Geometry check sheet. Reference: the model listing, model coordinates, mm. A direction names the side the tool comes from. Give positions to 0.01 mm unless a question says otherwise; leave off trailing zeros. Write each loop counter-clockwise with the first axis right and the second up, starting at its lowest first coordinate (ties: lowest second). Pieces come first, ordered by that corner, then holes.
(1) Depth check by flat-ended pin: P1, Ø5, axis at x = -40, z = -35, coming from the -Y side; P2, Ø6, axis at y = 19.5, z = -37.5, coming from the -X side; P3, Ø7, axis at x = 40, z = 35, coming from the +Y side. Enter the tip coordinate at first touch or a pass-through.
(2) Mould release check, pull along Z, two halves, no side actions. Record for faces 1 (the flat face through (-1, 15, 50)), 2 (the cylindrical face through (37.973, 1.521, 33.141)), 3 (the flat face through (-45, 1, -1)): +Z half, -Z half, draft (parallel to the pull), parting line (faces both ways), or undercut.
(3) Cross-section at D-D (x = 39). Record the boundary of the cut face in (y, z).
(4) Cross-section at B-B (z = -35). Record the boundary of the cut face in (x, y), and give its area (3 significant figures).
(5) Cross-section at C-C (z = -20.5). Record the boundary of the cut face in (x, y), and give its area (3 significant figures).
(6) Tool access check on faces 4 (the flat face through (35, 16, 1)), 5 (the cylindrical face through (-42.027, 1.521, 33.141)), 6 (the flat face through (-35, 16, 1)). Record the directions out of +Z, -Z, +X, -X, +Y, -Y that give a thin tool (end or side, any length) a straight path to the whole face; none if there is none.
(7) Cross-section at A-A (x = -40). Record the boundary of the cut face in (y, z), and give its area (3 significant figures).
(8) Thickness scan on line 1 along X through (y, z) = (1.8, -35); line 2 along Z through (x, y) = (-40, 1); line 3 along X through (y, z) = (21.75, -28). Record the ranges inside material, lowest first.
```python
from build123d import *

# Parameters (mm, degrees)
SKETCH1_W                = 70
SKETCH1_H                = 100
BOSS_EXTRUDE1_DEPTH      = 30
BOSS_EXTRUDE3_DEPTH      = 3
M5_CLEARANCE_SLOT1_D     = 5.5
M5_CLEARANCE_SLOT1_DEPTH = 22.25
M5_CLEARANCE_SLOT1_TIP   = 1.652366702


with BuildPart() as part:
    # Sketch1 → Boss-Extrude1 (new body)
    with BuildSketch(Plane(origin=(0, 0, 0), x_dir=(1, 0, 0), z_dir=(0, 1, 0))):
        Rectangle(SKETCH1_W, SKETCH1_H)
    extrude(amount=BOSS_EXTRUDE1_DEPTH)

    # Sketch1<4> → Boss-Extrude3 (add)
    with BuildSketch(Plane(origin=(0, 0, 0), x_dir=(1, 0, 0), z_dir=(0, 1, 0))):
        Polygon((-35, -50), (-35, 50), (-45, 50), (-45, 35), (-45, -35), (-45, -50), align=None)
        Polygon((45, 35), (45, 50), (35, 50), (35, -50), (45, -50), (45, -35), align=None)
    extrude(amount=BOSS_EXTRUDE3_DEPTH)

    # M5 Clearance Slot1
    with Locations(Plane(origin=(0, 0, 0), x_dir=(-1, 0, 0), z_dir=(0, -1, 0))):
        with Locations((40, 35), (40, -35), (-40, 35), (-40, -35)):
            Hole(M5_CLEARANCE_SLOT1_D / 2, depth=M5_CLEARANCE_SLOT1_DEPTH)
            with Locations((0, 0, -(M5_CLEARANCE_SLOT1_DEPTH + M5_CLEARANCE_SLOT1_TIP / 2))):  # 118° drill point
                Cone(0, M5_CLEARANCE_SLOT1_D / 2, M5_CLEARANCE_SLOT1_TIP, mode=Mode.SUBTRACT)


solid = part.part
```
Reply:
1. P1: passes through
1. P2: stops at x = -35
1. P3: stops at y = 3
2. face 1: +Z half
2. face 2: undercut
2. face 3: draft
3. outline: (0, -50) - (3, -50) - (3, -37.56) - (0, -37.56) - close; (0, -32.44) - (3, -32.44) - (3, 32.44) - (0, 32.44) - close; (0, 37.56) - (3, 37.56) - (3, 50) - (0, 50) - close
4. outline: (-45, 0) - (-42.75, 0) - (-42.75, 3) - (-45, 3) - close; (-37.25, 0) - (37.25, 0) - (37.25, 3) - (35, 3) - (35, 30) - (-35, 30) - (-35, 3) - (-37.25, 3) - close; (42.75, 0) - (45, 0) - (45, 3) - (42.75, 3) - close
4. area: 2,130 mm2
5. outline: (-45, 0) - (45, 0) - (45, 3) - (35, 3) - (35, 30) - (-35, 30) - (-35, 3) - (-45, 3) - close
5. area: 2,160 mm2
6. face 4: +Z, -Z, +X, +Y
6. face 5: +Y, -Y
6. face 6: +Z, -Z, -X, +Y
7. outline: (0, -50) - (3, -50) - (3, -37.75) - (0, -37.75) - close; (0, -32.25) - (3, -32.25) - (3, 32.25) - (0, 32.25) - close; (0, 37.75) - (3, 37.75) - (3, 50) - (0, 50) - close
7. area: 267 mm2
8. line 1: x = -45 to -42.75, -37.25 to 37.25, 42.75 to 45
8. line 2: z = -50 to -37.75, -32.25 to 32.25, 37.75 to 50
8. line 3: x = -35 to 35
